Autodesk Inventor part; units mm, degrees
ref_plane "YZ Plane" through (0, 0, 0) normal (1, 0, 0) x (0, 1, 0)
ref_plane "XZ Plane" through (0, 0, 0) normal (0, 1, 0) x (-1, 0, 0)
ref_plane "XY Plane" through (0, 0, 0) normal (0, 0, 1) x (1, 0, 0)
sketch "草圖1" plane through (0, 0, 0) normal (0, 0, 1) x (1, 0, 0)
  arc A0 (-17.0574, -3.0077) -> (5.924, 16.276) centre (-22.2668, 26.5366) ccw
  line L0 (5.924, 16.276) -> (41.0424, 112.7631)
  line L1 (-118.1769, -20.8378) -> (-17.0574, -3.0077)
  line L2 (-118.1769, -20.8378) -> (-26.5575, -28.8534)
  arc A1 (-26.5575, -28.8534) -> (33.0268, 21.1437) centre (-21.764, 25.9373) ccw
  line L3 (33.0268, 21.1437) -> (41.0424, 112.7631)
  circle A2 centre (7.3253, -8.7299) radius 2
  point P0 (0, 0)
  dimension "d0" = 55
  dimension "d1" = 4
  dimension "d2" = 23
  dimension "d3" = 23
extrude "擠出1" add sketch "草圖1" along normal blind 3
sketch "草圖2" plane through (0, 0, 3) normal (0, 0, 1) x (1, 0, 0)
  arc A0 (-26.5575, -28.8534) -> (33.0268, 21.1437) centre (-21.764, 25.9373) ccw
  line L0 (33.0268, 21.1437) -> (41.0424, 112.7631)
  line L1 (41.0424, 112.7631) -> (5.924, 16.276)
  arc A1 (-17.0574, -3.0077) -> (5.924, 16.276) centre (-22.2668, 26.5366) ccw
  line L2 (-17.0574, -3.0077) -> (-118.1769, -20.8378)
  line L3 (-118.1769, -20.8378) -> (-26.5575, -28.8534)
  circle A2 centre (7.3253, -8.7299) radius 2
  point P0 (0, 0)
equation "\"d3\" = d2"
properties part number "sus_1"
Geometry: final body of the model. Coordinates: model frame, mm. Round coordinates to 2 decimals unless told otherwise and drop trailing zeros. Write each loop counter-clockwise with the first axis right and the second up, starting at its lowest first coordinate (ties: lowest second). Pieces come first, ordered by that corner, then holes.
Item 1: Section query C-C (x = -75). Return loops of the section in (y, z), plus the area to 3 significant figures.
Item 2: Pin query (flat end, axial travel): P1, Ø4.5, axis at x = 7.33, y = -8.73, coming from the +Z side. Return the tip coordinate at first contact, or that it passes through.
Item 3: Material intervals for L1, parallel to X at y = 39, z = 2.3; L2, parallel to Y at x = -41.5, z = 2.45; L3, parallel to X at y = 2.5, z = 1.45, sorted ascending.
Item 4: Section query A-A (z = 1.85). Return loops of the section in (x, y), plus the area to 3 significant figures.
Item 5: Mould query, pull axis X, two halves, no side actions, for faces 1 (the face through (-68.325, -12.048, 1.479)), 2 (the face through (9.233, -9.331, 1.479)), 3 (the face through (36.98, 66.31, 1.48)), 4 (the face through (-9, -5, 3)). Classes: +X half, -X half, draft (parallel to the pull), parting line (faces both ways), or undercut.
Item 6: Section query B-B (y = 102). Return loops of the section in (x, z).
Completed:
1. outline: (-24.62, 0) - (-13.22, 0) - (-13.22, 3) - (-24.62, 3) - close
1. area: 34.2 mm2
2. P1: stops at z = 3
3. L1: x = 14.19 to 34.59
3. L2: y = -27.55 to -7.32
3. L3: x = -4.32 to 27.99
4. outline: (-118.18, -20.84) - (-26.56, -28.85) arc R55 ccw to (33.03, 21.14) - (41.04, 112.76) - (5.92, 16.28) arc R30 cw to (-17.06, -3.01) - close; hole circle Ø4 at (7.33, -8.73)
4. area: 3,950 mm2
5. face 1: -X half
5. face 2: undercut
5. face 3: +X half
5. face 4: draft
6. outline: (37.12, 0) - (40.1, 0) - (40.1, 3) - (37.12, 3) - close
